Build history of the part. All positions in model axes, mm. A direction names the side the tool comes from. Give positions to 0.01 mm unless a question says otherwise; leave off trailing zeros. Write each loop counter-clockwise with the first axis right and the second up, starting at its lowest first coordinate (ties: lowest second). Pieces come first, ordered by that corner, then holes. Notation, with made-up numbers: (88, 49.5) -> (100, 49.5) arc R22 ccw to (100, 72.5) -> close; hole circle Ø1 at (27.25, 5.25). An arc over 180 degrees is marked (long way). Write item = value, one per line. Start each with the question number.
Q1. Saw through at A-A, the plane x = 0. List the corners of the cut face in (y, z), then the cut area to 3 significant figures.
Q2. Drop flat-ended pins along their axis: P1, Ø2, axis at x = 8.5, y = 0, coming from the -Z side; P2, Ø0.6, axis at x = 8, y = -0.5, coming from the +Z side; P3, Ø3.5, axis at x = 12, z = 2, coming from the -Y side. Give the stop position or say it passes through.
Q3. Mould opens along Z. For faces 4 (the face through (7, -1, 2)), 5 (the face through (11, 0, 0)), 6 (the face through (0, -3, 1)), 7 (the face through (10, -2, 1)) say: pulls with the +Z half, pulls with the -Z half, needs draft (parallel to the pull), parting line crosses it, or undercut.
Q4. Saw through at B-B, the plane y = -0.75. List the corners of the cut face in (x, z), then the cut area to 3 significant figures.
Q5. Saw through at D-D, the plane y = 0.75. List the corners of the cut face in (x, z).
Q6. Tool access for faces 1 (the face through (1, 0, -1)), 2 (the face through (4.9, -3.5, 1)), 3 (the face through (10, 1, 1)): list every direction of +Z, -Z, +X, -X, +Y, -Y with a clear straight run to the whole face (end or side of a thin tool).
Q7. Wall check: line 1 (Z direction, x = 0, y = -1.2); line 2 (Y direction, x = -0.25, z = -3.5); line 3 (X direction, y = -0.5, z = -0.5). Give the ranges that are in metal, low to high.
Q8. Saw through at C-C, the plane z = -0.75. List the corners of the cut face in (x, y), then the cut area to 3 significant figures.
from build123d import *

# Parameters (mm, degrees)
F1_DEPTH = 5
F2_DEPTH = 2
F3_DEPTH = 2
F4_D     = 2
F5_R     = 1


with BuildPart() as f1:
    # F0 (on Front) → F1 (new body)
    with BuildSketch(Plane.XZ):
        with BuildLine():
            ThreePointArc((4.582576, 2), (-4.894532, -1.021548), (5, 0))
            ThreePointArc((5, 0), (4.894532, 1.021548), (4.582576, 2))
        make_face()
    extrude(amount=F1_DEPTH)

    # F0 (on Front) → F2 (join)
    with BuildSketch(Plane.XZ):
        with BuildLine():
            ThreePointArc((4.582576, 2), (4.894532, 1.021548), (5, 0))
            Line((5, 0), (10, 0))
            Line((10, 0), (10, 2))
            Line((10, 2), (4.582576, 2))
        make_face()
    extrude(amount=F2_DEPTH)

    # F0 (on Front) → F3 (join, symmetric)
    with BuildSketch(Plane.XZ):
        Polygon((10, 2), (10, 0), (15.196152, 0), (15.196152, 1), (10, 4), align=None)
    extrude(amount=F3_DEPTH, both=True)

    # F4 (through all)
    with Locations(Plane(origin=(0, 0, 0), x_dir=(1, 0, 0), z_dir=(0, 1, 0))):
        with Locations((0, 0)):
            Hole(F4_D / 2)

    # F5
    f5_edges = [f1.edges().sort_by_distance(p)[0] for p in [
        (10, 0, 4),
    ]]
    fillet(f5_edges, radius=F5_R)


solid = f1.part
Report:
q1.outline = (-5, -5) -> (0, -5) -> (0, -1) -> (-5, -1) -> close; (-5, 1) -> (0, 1) -> (0, 5) -> (-5, 5) -> close
q1.area = 40.0 mm2
q2.P1 = 0
q2.P2 = 2
q2.P3 = -2
q3.face_4 = pulls with the +Z half
q3.face_5 = pulls with the -Z half
q3.face_6 = undercut
q3.face_7 = needs draft
q4.outline = (4.58, 2) arc R5 ccw (long way) to (5, 0) -> (15.2, 0) -> (15.2, 1) -> (11.5, 3.13) arc R1 ccw to (10, 2.27) -> (10, 2) -> close; hole circle Ø2 at (0, 0)
q4.area = 98.0 mm2
q5.outline = (10, 0) -> (15.2, 0) -> (15.2, 1) -> (11.5, 3.13) arc R1 ccw to (10, 2.27) -> close
q6.face_1 = +Z, -Z, -X, +Y
q6.face_2 = +Z, +X, -Y
q6.face_3 = +Z, +Y
q7.line_1 = -5 to -1, 1 to 5
q7.line_2 = -5 to 0
q7.line_3 = -4.97 to -0.87, 0.87 to 4.97
q8.outline = (-4.94, -5) -> (-0.66, -5) -> (-0.66, 0) -> (-4.94, 0) -> close; (0.66, -5) -> (4.94, -5) -> (4.94, 0) -> (0.66, 0) -> close
q8.area = 42.8 mm2
